Work out the finished part from the listing and answer in its coordinate system (mm). Face numbers are marked on the shaded views. A direction names the side the tool comes from. Round coordinates to 2 decimals unless told otherwise and drop trailing zeros. Write each loop counter-clockwise with the first axis right and the second up, starting at its lowest first coordinate (ties: lowest second). Pieces come first, ordered by that corner, then holes.
1. Determine the mould class of the marked faces 1, 2 and 3 for opening direction Z: pulls with the +Z half, pulls with the -Z half, needs draft (parallel to the pull), parting line crosses it, or undercut.
2. Find section A-A (z = -9.5). Write down the section's boundary in (x, y), and give its area (3 significant figures).
3. Find section C-C (z = -13). Write down the section's boundary in (x, y), and give its area (3 significant figures).
4. Flat-ended cylindrical pins translate along their axes: pin 1 Ø0.7 at (y, z) = (1.5, -6.5) entering from +X; pin 2 Ø1.1 at (x, y) = (16.5, 2) entering from +Z; pin 3 Ø0.8 at (x, z) = (10.5, -19) entering from -Y. Find the tip coordinate at first contact, or state that the pin passes through.
5. A tool of negligible diameter and unlimited length cuts with its end or side. For the marked faces 4, 5 and 6, from which of +Z, -Z, +X, -X, +Y, -Y can it reach the whole face along a straight path? Write none if from no direction.
6. Find section B-B (x = 27.5). Write down the section's boundary in (y, z) (3 decimals), and give its area (3 significant figures).
7. Find section D-D (x = 22.5). Write down the section's boundary in (y, z) (3 decimals).
8. Straight lines are drawn through the part: probe 1 along X at (y, z) = (3, 2.5); probe 2 along X at (y, z) = (3.25, -1.25); probe 3 along Z at (x, y) = (25, 3) (3 decimals). For each, find the intervals that lie inside material, in ascending order.
```python
from build123d import *

# Parameters (mm, degrees)
SKETCH1_W           = 35.4
SKETCH1_H           = 25.65
SKETCH1_R           = 2.125
BOSS_EXTRUDE1_DEPTH = 2
SKETCH1_3_R         = 2.125
BOSS_EXTRUDE2_DEPTH = 6
SKETCH2_W           = 3
SKETCH2_H           = 4.5
CUT_EXTRUDE1_DEPTH  = 5
CHAMFER1_SIZE       = 1.5
FILLET1_R           = 1
SKETCH3_W           = 7
SKETCH3_H           = 5.470677448
CUT_EXTRUDE2_DEPTH  = 6
SKETCH4_R           = 1
CUT_EXTRUDE3_DEPTH  = 2
SKETCH5_W           = 10
SKETCH5_H           = 1.310302081
BOSS_EXTRUDE3_DEPTH = 1
FILLET2_R           = 1.5


with BuildPart() as part:
    # Sketch1 → Boss-Extrude1 (new body)
    with BuildSketch(Plane(origin=(0, 0, 0), x_dir=(1, 0, 0), z_dir=(0, 1, 0))):
        with Locations((16.5, 7)):
            Rectangle(SKETCH1_W, SKETCH1_H)
        with Locations(Location((30.875, -2.5, 0), (0, 0, 270))):
            Circle(SKETCH1_R, mode=Mode.SUBTRACT)
        with Locations(Location((2.125, -2.5, 0), (0, 0, 270))):
            Circle(SKETCH1_R, mode=Mode.SUBTRACT)
        with Locations(Location((2.125, 16.5, 0), (0, 0, 270))):
            Circle(SKETCH1_R, mode=Mode.SUBTRACT)
        with Locations(Location((30.875, 16.5, 0), (0, 0, 270))):
            Circle(SKETCH1_R, mode=Mode.SUBTRACT)
    extrude(amount=BOSS_EXTRUDE1_DEPTH)

    # Sketch1<3> → Boss-Extrude2 (add)
    # profile 1 of 2: a face of its own
    with BuildSketch(Plane(origin=(0, 0, 0), x_dir=(1, 0, 0), z_dir=(0, 1, 0))):
        Polygon((33, 0), (0, 0), (0, 2), (-1.2, 2), (-1.2, -5.825), (34.2, -5.825), (34.2, 3.5), (33, 3.5), align=None)
        with Locations(Location((2.125, -2.5, 0), (0, 0, 270))):
            Circle(SKETCH1_3_R, mode=Mode.SUBTRACT)
        with Locations(Location((30.875, -2.5, 0), (0, 0, 270))):
            Circle(SKETCH1_3_R, mode=Mode.SUBTRACT)
    # profile 2 of 2: a face of its own
    with BuildSketch(Plane(origin=(0, 0, 0), x_dir=(1, 0, 0), z_dir=(0, 1, 0))):
        Polygon((-1.2, 12), (0, 12), (0, 14), (33, 14), (33, 10.5), (34.2, 10.5), (34.2, 19.825), (-1.2, 19.825), align=None)
        with Locations(Location((2.125, 16.5, 0), (0, 0, 270))):
            Circle(SKETCH1_3_R, mode=Mode.SUBTRACT)
        with Locations(Location((30.875, 16.5, 0), (0, 0, 270))):
            Circle(SKETCH1_3_R, mode=Mode.SUBTRACT)
    extrude(amount=BOSS_EXTRUDE2_DEPTH)

    # Sketch2 → Cut-Extrude1 (cut)
    with BuildSketch(Plane(origin=(0, 0, 0), x_dir=(-1, 0, 0), z_dir=(0, -1, 0))):
        with Locations((-10.5, -3.575)):
            Rectangle(SKETCH2_W, SKETCH2_H)
        with Locations((-16.5, -3.575)):
            Rectangle(SKETCH2_W, SKETCH2_H)
        with Locations((-22.5, -3.575)):
            Rectangle(SKETCH2_W, SKETCH2_H)
        with Locations((-22.5, 17.575)):
            Rectangle(SKETCH2_W, SKETCH2_H)
        with Locations((-16.5, 17.575)):
            Rectangle(SKETCH2_W, SKETCH2_H)
        with Locations((-10.5, 17.575)):
            Rectangle(SKETCH2_W, SKETCH2_H)
    extrude(amount=-CUT_EXTRUDE1_DEPTH, mode=Mode.SUBTRACT)

    # Chamfer1
    # the kernel refuses this chamfer: 1.5 mm, written as the material it adds along each edge
    with BuildSketch(Plane(origin=(5.142475518, 5, -15.325), x_dir=(0, -0.9996219169112968, 0.027495876610586775), z_dir=(1, 0, 0)), Plane(origin=(11.142475518, 5, -15.325), x_dir=(0, -0.9996219169112968, 0.027495876610586775), z_dir=(1, 0, 0)), Plane(origin=(17.142475518, 5, -15.325), x_dir=(0, -0.9996219169112968, 0.027495876610586775), z_dir=(1, 0, 0)), Plane(origin=(5.142475518, 5, 1.325), x_dir=(0, 0.0274958766105862, 0.9996219169112968), z_dir=(1, 0, 0))) as chamfer1_piece_1:
        Polygon((CHAMFER1_SIZE * 0.999621916911, CHAMFER1_SIZE * 0.0274958766106), (-CHAMFER1_SIZE * 0.0274958766106, CHAMFER1_SIZE * 0.999621916911), (0, 0), align=None)
    extrude(amount=10.715048964)
    with BuildSketch(Plane(origin=(27.857524482, 5, 1.325), x_dir=(0, 0.0274958766105862, 0.9996219169112968), z_dir=(-1, 0, 0)), Plane(origin=(21.857524482, 5, 1.325), x_dir=(0, 0.0274958766105862, 0.9996219169112968), z_dir=(-1, 0, 0))) as chamfer1_piece_2:
        Polygon((CHAMFER1_SIZE * 0.999621916911, -CHAMFER1_SIZE * 0.0274958766106), (-CHAMFER1_SIZE * 0.0274958766106, -CHAMFER1_SIZE * 0.999621916911), (0, 0), align=None)
    extrude(amount=10.715048964)
    # the kernel refuses this chamfer: 1.5 mm, written as the material it takes off along each edge
    with BuildSketch(Plane(origin=(18.857524482, 0, -19.825), x_dir=(0, 0.9996219169112968, -0.027495876610586778), z_dir=(-1, 0, 0)), Plane(origin=(24.857524482, 0, -19.825), x_dir=(0, 0.9996219169112968, -0.027495876610586778), z_dir=(-1, 0, 0)), Plane(origin=(8.142475518, 0, 5.825), x_dir=(0, 0.9996219169112968, 0.027495876610586202), z_dir=(1, 0, 0)), Plane(origin=(14.142475518, 0, 5.825), x_dir=(0, 0.9996219169112968, 0.027495876610586202), z_dir=(1, 0, 0))) as chamfer1_2_piece_1:
        Polygon((CHAMFER1_SIZE * 0.999621916911, -CHAMFER1_SIZE * 0.0274958766106), (-CHAMFER1_SIZE * 0.0274958766106, -CHAMFER1_SIZE * 0.999621916911), (0, 0), align=None)
    extrude(amount=10.715048964, mode=Mode.SUBTRACT)
    with BuildSketch(Plane(origin=(38.057524482, 0, -19.825), x_dir=(0, 0.9996219169112968, -0.027495876610586778), z_dir=(-1, 0, 0)), Plane(origin=(20.142475518, 0, 5.825), x_dir=(0, 0.9996219169112968, 0.027495876610586202), z_dir=(1, 0, 0)), Plane(origin=(-5.057524482, 0, 5.825), x_dir=(0, 0.9996219169112968, 0.027495876610586202), z_dir=(1, 0, 0)), Plane(origin=(12.857524482, 0, -19.825), x_dir=(0, 0.9996219169112968, -0.027495876610586778), z_dir=(-1, 0, 0))) as chamfer1_2_piece_2:
        Polygon((CHAMFER1_SIZE * 0.999621916911, -CHAMFER1_SIZE * 0.0274958766106), (-CHAMFER1_SIZE * 0.0274958766106, -CHAMFER1_SIZE * 0.999621916911), (0, 0), align=None)
    extrude(amount=17.915048964, mode=Mode.SUBTRACT)

    # Fillet1
    # the kernel refuses this fillet: 1 mm, written as the material it adds along each edge
    with BuildSketch(Plane(origin=(21, 0, -15.325), x_dir=(0, 0, -1), z_dir=(0, 1, 0)), Plane(origin=(15, 0, -15.325), x_dir=(0, 0, -1), z_dir=(0, 1, 0)), Plane(origin=(12, 0, -15.325), x_dir=(-1, 0, 0), z_dir=(0, 1, 0)), Plane(origin=(24, 0, -15.325), x_dir=(-1, 0, 0), z_dir=(0, 1, 0)), Plane(origin=(18, 0, -15.325), x_dir=(-1, 0, 0), z_dir=(0, 1, 0)), Plane(origin=(12, 0, 1.325), x_dir=(0, 0, 1), z_dir=(0, 1, 0)), Plane(origin=(18, 0, 1.325), x_dir=(0, 0, 1), z_dir=(0, 1, 0)), Plane(origin=(9, 0, 1.325), x_dir=(1, 0, 0), z_dir=(0, 1, 0)), Plane(origin=(15, 0, 1.325), x_dir=(1, 0, 0), z_dir=(0, 1, 0)), Plane(origin=(21, 0, 1.325), x_dir=(1, 0, 0), z_dir=(0, 1, 0))) as fillet1_piece_1:
        with BuildLine():
            CenterArc((FILLET1_R, -FILLET1_R), FILLET1_R, 90, 90)
            Line((0, -FILLET1_R), (0, 0))
            Line((0, 0), (FILLET1_R, 0))
        make_face()
    extrude(amount=6)
    with BuildSketch(Plane(origin=(21, 5, -19.825), x_dir=(1, 0, 0), z_dir=(0, 0, 1)), Plane(origin=(15, 5, -19.825), x_dir=(1, 0, 0), z_dir=(0, 0, 1)), Plane(origin=(9, 5, -19.825), x_dir=(1, 0, 0), z_dir=(0, 0, 1)), Plane(origin=(12, 5, -14.325), x_dir=(-1, 0, 0), z_dir=(0, 0, -1)), Plane(origin=(24, 5, -14.325), x_dir=(-1, 0, 0), z_dir=(0, 0, -1)), Plane(origin=(18, 5, -14.325), x_dir=(-1, 0, 0), z_dir=(0, 0, -1)), Plane(origin=(15, 5, 0.325), x_dir=(1, 0, 0), z_dir=(0, 0, 1)), Plane(origin=(24, 5, 5.825), x_dir=(-1, 0, 0), z_dir=(0, 0, -1)), Plane(origin=(18, 5, 5.825), x_dir=(-1, 0, 0), z_dir=(0, 0, -1))) as fillet1_piece_2:
        with BuildLine():
            CenterArc((FILLET1_R, -FILLET1_R), FILLET1_R, 90, 90)
            Line((0, -FILLET1_R), (0, 0))
            Line((0, 0), (FILLET1_R, 0))
        make_face()
    extrude(amount=5.5)
    with BuildSketch(Plane(origin=(9, 0, -15.325), x_dir=(1, 0, 0), z_dir=(0, 1, 0)), Plane(origin=(24, 0, 1.325), x_dir=(-1, 0, 0), z_dir=(0, 1, 0))) as fillet1_piece_3:
        with BuildLine():
            CenterArc((FILLET1_R, FILLET1_R), FILLET1_R, 180, 90)
            Line((0, FILLET1_R), (0, 0))
            Line((0, 0), (FILLET1_R, 0))
        make_face()
    extrude(amount=6)
    with BuildSketch(Plane(origin=(21, 5, 0.325), x_dir=(0, -1, 0), z_dir=(0, 0, 1)), Plane(origin=(9, 5, 5.825), x_dir=(1, 0, 0), z_dir=(0, 0, -1)), Plane(origin=(12, 5, 0.325), x_dir=(-1, 0, 0), z_dir=(0, 0, 1))) as fillet1_piece_4:
        with BuildLine():
            CenterArc((FILLET1_R, FILLET1_R), FILLET1_R, 180, 90)
            Line((0, FILLET1_R), (0, 0))
            Line((0, 0), (FILLET1_R, 0))
        make_face()
    extrude(amount=5.5)
    # the kernel refuses this fillet: 1 mm, written as the material it takes off along each edge
    with BuildSketch(Plane(origin=(35.235533906, 0, -18.325), x_dir=(0, 0, 1), z_dir=(-1, 0, 0)), Plane(origin=(2.071956853, 0, -18.325), x_dir=(0, 0, 1), z_dir=(-1, 0, 0)), Plane(origin=(-2.235533906, 0, 4.325), x_dir=(0, 0, -1), z_dir=(1, 0, 0)), Plane(origin=(30.928043147, 0, 4.325), x_dir=(0, 0, -1), z_dir=(1, 0, 0))) as fillet1_2_piece_1:
        with BuildLine():
            CenterArc((FILLET1_R * 0.414213562373, FILLET1_R), FILLET1_R, 225, 45)
            Line((-FILLET1_R * 0.292893218813, FILLET1_R * 0.292893218813), (0, 0))
            Line((0, 0), (FILLET1_R * 0.414213562373, 0))
        make_face()
    extrude(amount=4.307490759, mode=Mode.SUBTRACT)
    with BuildSketch(Plane(origin=(22.964466094, 1.5, -19.825), x_dir=(0, -0.7071067811862655, 0.7071067811868295), z_dir=(1, 0, 0)), Plane(origin=(-2.235533906, 1.5, -19.825), x_dir=(0, -0.7071067811862655, 0.7071067811868295), z_dir=(1, 0, 0))) as fillet1_2_piece_2:
        with BuildLine():
            CenterArc((FILLET1_R * 0.414213562373, -FILLET1_R), FILLET1_R, 90, 45)
            Line((-FILLET1_R * 0.292893218814, -FILLET1_R * 0.292893218814), (0, 0))
            Line((0, 0), (FILLET1_R * 0.414213562373, 0))
        make_face()
    extrude(amount=12.271067812, mode=Mode.SUBTRACT)
    with BuildSketch(Plane(origin=(22.964466094, 0, -18.325), x_dir=(0, 0, 1), z_dir=(1, 0, 0)), Plane(origin=(2.178043147, 0, -18.325), x_dir=(0, 0, 1), z_dir=(1, 0, 0)), Plane(origin=(10.035533906, 0, 4.325), x_dir=(0, 0, -1), z_dir=(-1, 0, 0)), Plane(origin=(30.821956853, 0, 4.325), x_dir=(0, 0, -1), z_dir=(-1, 0, 0))) as fillet1_2_piece_3:
        with BuildLine():
            CenterArc((FILLET1_R * 0.414213562373, -FILLET1_R), FILLET1_R, 90, 45)
            Line((-FILLET1_R * 0.292893218813, -FILLET1_R * 0.292893218813), (0, 0))
            Line((0, 0), (FILLET1_R * 0.414213562373, 0))
        make_face()
    extrude(amount=7.857490759, mode=Mode.SUBTRACT)
    with BuildSketch(Plane(origin=(16.964466094, 1.5, -19.825), x_dir=(0, -0.7071067811862655, 0.7071067811868295), z_dir=(1, 0, 0)), Plane(origin=(16.964466094, 0, -18.325), x_dir=(0, 0, 1), z_dir=(1, 0, 0)), Plane(origin=(10.964466094, 1.5, -19.825), x_dir=(0, -0.7071067811862655, 0.7071067811868295), z_dir=(1, 0, 0)), Plane(origin=(10.964466094, 0, -18.325), x_dir=(0, 0, 1), z_dir=(1, 0, 0)), Plane(origin=(16.035533906, 0, 4.325), x_dir=(0, 0, -1), z_dir=(-1, 0, 0)), Plane(origin=(22.035533906, 0, 4.325), x_dir=(0, 0, -1), z_dir=(-1, 0, 0))) as fillet1_2_piece_4:
        with BuildLine():
            CenterArc((FILLET1_R * 0.414213562373, -FILLET1_R), FILLET1_R, 90, 45)
            Line((-FILLET1_R * 0.292893218814, -FILLET1_R * 0.292893218814), (0, 0))
            Line((0, 0), (FILLET1_R * 0.414213562373, 0))
        make_face()
    extrude(amount=5.071067812, mode=Mode.SUBTRACT)
    with BuildSketch(Plane(origin=(-2.235533906, 1.5, 5.825), x_dir=(0, -0.707106781186265, -0.70710678118683), z_dir=(1, 0, 0)), Plane(origin=(22.964466094, 1.5, 5.825), x_dir=(0, -0.707106781186265, -0.70710678118683), z_dir=(1, 0, 0))) as fillet1_2_piece_5:
        with BuildLine():
            CenterArc((FILLET1_R * 0.414213562373, FILLET1_R), FILLET1_R, 225, 45)
            Line((-FILLET1_R * 0.292893218814, FILLET1_R * 0.292893218814), (0, 0))
            Line((0, 0), (FILLET1_R * 0.414213562373, 0))
        make_face()
    extrude(amount=12.271067812, mode=Mode.SUBTRACT)
    with BuildSketch(Plane(origin=(10.964466094, 1.5, 5.825), x_dir=(0, -0.7071067811862647, -0.7071067811868302), z_dir=(1, 0, 0)), Plane(origin=(16.964466094, 1.5, 5.825), x_dir=(0, -0.7071067811862652, -0.7071067811868297), z_dir=(1, 0, 0))) as fillet1_2_piece_6:
        with BuildLine():
            CenterArc((FILLET1_R * 0.414213562373, FILLET1_R), FILLET1_R, 225, 45)
            Line((-FILLET1_R * 0.292893218814, FILLET1_R * 0.292893218814), (0, 0))
            Line((0, 0), (FILLET1_R * 0.414213562373, 0))
        make_face()
    extrude(amount=5.071067812, mode=Mode.SUBTRACT)

    # Sketch3 → Cut-Extrude2 (cut)
    with BuildSketch(Plane(origin=(34.2, 0, 0), x_dir=(0, 0, -1), z_dir=(1, 0, 0))):
        with Locations((7, 3.264661276)):
            Rectangle(SKETCH3_W, SKETCH3_H)
    extrude(amount=-CUT_EXTRUDE2_DEPTH, mode=Mode.SUBTRACT)

    # Sketch4 → Cut-Extrude3 (cut)
    with BuildSketch(Plane(origin=(0, 2, 0), x_dir=(1, 0, 0), z_dir=(0, 1, 0))):
        with Locations(Location((9.446942501, 11.641698117, 0), (0, 0, 270))):
            Circle(SKETCH4_R)
        with Locations(Location((30.446985681, 11.641698117, 0), (0, 0, 270))):
            Circle(SKETCH4_R)
        with Locations(Location((30.446985681, 2.141677797, 0), (0, 0, 270))):
            Circle(SKETCH4_R)
    extrude(amount=-CUT_EXTRUDE3_DEPTH, mode=Mode.SUBTRACT)

    # Sketch5 → Boss-Extrude3 (add)
    with BuildSketch(Plane.ZY.offset(1.2)):
        with Locations((-7, 2.65515104)):
            Rectangle(SKETCH5_W, SKETCH5_H)
    extrude(amount=-BOSS_EXTRUDE3_DEPTH)

    # Fillet2
    fillet2_edges = [part.edges().sort_by_distance(p)[0] for p in [
        (-0.7, 3.310302081, -12),
        (-0.7, 3.310302081, -2),
    ]]
    fillet(fillet2_edges, radius=FILLET2_R)


solid = part.part
```
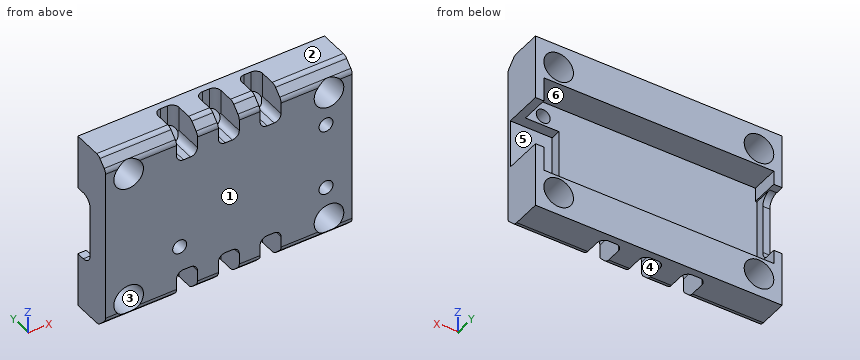
Worked answers:
1. face 1: needs draft
1. face 2: pulls with the +Z half
1. face 3: undercut
2. outline: (-1.2, 0) - (34.2, 0) - (34.2, 0.53) - (28.2, 0.53) - (28.2, 2) - (-0.2, 2) - (-0.2, 3.31) - (-1.2, 3.31) - close
2. area: 63.3 mm2
3. outline: (-1.2, 0) - (34.2, 0) - (34.2, 6) - (33, 6) - (33, 2) - (0, 2) - (0, 6) - (-1.2, 6) - close
3. area: 80.4 mm2
4. pin 1: stops at x = 28.2
4. pin 2: stops at z = 1.33
4. pin 3: stops at y = 5
5. face 4: -Z, -Y
5. face 5: +X, +Y
5. face 6: +Y
6. outline: (0, -17.911) arc R1 ccw to (0.293, -18.618) - (1.207, -19.532) arc R1 ccw to (1.914, -19.825) - (6, -19.825) - (6, -14) - (2, -14) - (2, 0) - (6, 0) - (6, 5.825) - (1.914, 5.825) arc R1 ccw to (1.207, 5.532) - (0.293, 4.618) arc R1 ccw to (0, 3.911) - close
6. area: 95.6 mm2
7. outline: (0, -15.325) - (3.5, -15.325) - (5, -16.825) - (5, -19.825) - (6, -19.825) - (6, -14) - (2, -14) - (2, 0) - (6, 0) - (6, 5.825) - (5, 5.825) - (5, 2.825) - (3.5, 1.325) - (0, 1.325) - close
8. probe 1: x = -1.2 to 0, 4.25 to 9, 12 to 15, 18 to 21, 24 to 28.75, 33 to 34.2
8. probe 2: x = -1.2 to 0, 33 to 34.2
8. probe 3: z = -19.825 to -14, 0 to 5.825
